from build123d import *

# Parameters (mm, degrees)
SKETCH1_W                    = 190
SKETCH1_H                    = 110
BASE_FLANGE1_DEPTH           = 1
EDGE_FLANGE1_START           = -72
EDGE_FLANGE1_DEPTH           = 144
EDGE_FLANGE2_STRIP_W         = 5.4732
EDGE_FLANGE2_STRIP_H         = 1
EDGE_FLANGE2_STRIP_CUT_DEPTH = 110
EDGE_FLANGE2_DEPTH           = 110
EDGE_FLANGE3_DEPTH           = 188.5268
SKETCH17_R                   = 2.25
SKETCH17_W                   = 10
SKETCH17_H                   = 25
CUT_EXTRUDE1_DEPTH           = 115.427372832
SKETCH18_R                   = 2.25
CUT_EXTRUDE2_DEPTH           = 115.427372832


# Read off the part's stored shape, not the designer's step: Edge-Flange1
# Sheet-metal steps are written as plain solids
with BuildPart() as part:
    # Sketch1 → Base-Flange1 (new body)
    with BuildSketch(Plane(origin=(0, 0, 0), x_dir=(1, 0, 0), z_dir=(0, 1, 0))):
        Rectangle(SKETCH1_W, SKETCH1_H)
    extrude(amount=-BASE_FLANGE1_DEPTH)

    # Edge-Flange1 outline → Edge-Flange1 (add)
    with BuildSketch(Plane.YZ.offset(EDGE_FLANGE1_START)):
        with BuildLine():
            Line((-11, -57.7366), (-1.7366, -57.7366))
            ThreePointArc((-1.7366, -57.7366), (-0.508638364, -57.227961636), (0, -56))
            Line((0, -56), (0, -55))
            Line((0, -55), (-1, -55))
            Line((-1, -55), (-1, -56))
            ThreePointArc((-1, -56), (-1.215745145, -56.520854855), (-1.7366, -56.7366))
            Line((-1.7366, -56.7366), (-11, -56.7366))
            Line((-11, -56.7366), (-11, -57.7366))
        make_face()
    extrude(amount=EDGE_FLANGE1_DEPTH)

    # Edge-Flange2 strip (across the edge) → Edge-Flange2 strip cut (cut)
    with BuildSketch(Plane(origin=(-95, -1, 55), x_dir=(1, 0, 0), z_dir=(0, 0, -1))):
        with Locations((-2, -0.5)):
            Rectangle(EDGE_FLANGE2_STRIP_W, EDGE_FLANGE2_STRIP_H)
    edge_flange2_strip_cut = extrude(amount=EDGE_FLANGE2_STRIP_CUT_DEPTH, mode=Mode.SUBTRACT)

    # Edge-Flange2 section (across the edge) → Edge-Flange2 (add)
    with BuildSketch(Plane(origin=(-95, -1, 55), x_dir=(1, 0, 0), z_dir=(0, 0, -1))):
        with BuildLine():
            Line((-1, 0.7366), (-1, 10))
            Line((-1, 10), (0, 10))
            Line((0, 10), (0, 0.7366))
            ThreePointArc((0, 0.7366), (0.215745145, 0.215745145), (0.7366, 0))
            Line((0.7366, 0), (0.7366, -1))
            ThreePointArc((0.7366, -1), (-0.491361636, -0.491361636), (-1, 0.7366))
        make_face()
    edge_flange2 = extrude(amount=EDGE_FLANGE2_DEPTH)

    # Mirror1: Edge-Flange2 strip cut, Edge-Flange2 across plane
    add(edge_flange2_strip_cut.mirror(Plane(origin=(0, 0, 0), x_dir=(0, 0, 1), z_dir=(1, 0, 0))), mode=Mode.SUBTRACT)
    add(edge_flange2.mirror(Plane(origin=(0, 0, 0), x_dir=(0, 0, 1), z_dir=(1, 0, 0))))

    # Edge-Flange3 section (across the edge) → Edge-Flange3 (add)
    with BuildSketch(Plane(origin=(94.2634, -1, 55.425276208), x_dir=(0, -0.5000000000000041, -0.8660254037844364), z_dir=(-1, 0, 0))):
        with BuildLine():
            Line((-1, 0.425276208), (-1, 10))
            Line((-1, 10), (0, 10))
            Line((0, 10), (0, 0.425276208))
            ThreePointArc((0, 0.425276208), (0.098685688, 0.056976208), (0.3683, -0.212638104))
            Line((0.3683, -0.212638104), (-0.1317, -1.078663508))
            ThreePointArc((-0.1317, -1.078663508), (-0.767339716, -0.443023792), (-1, 0.425276208))
        make_face()
    extrude(amount=EDGE_FLANGE3_DEPTH)

    # Sketch17 → Cut-Extrude1 (cut, through all)
    with BuildSketch(Plane(origin=(0, 0, 0), x_dir=(1, 0, 0), z_dir=(0, 1, 0))):
        with Locations(Location((66, 0, 0), (0, 0, 270))):
            Circle(SKETCH17_R)
        with Locations(Location((55, 0, 0), (0, 0, 270))):
            Circle(SKETCH17_R)
        with Locations(Location((-55, 0, 0), (0, 0, 270))):
            Circle(SKETCH17_R)
        with Locations(Location((-66, 0, 0), (0, 0, 270))):
            Circle(SKETCH17_R)
        with Locations((79, 0)):
            Rectangle(SKETCH17_W, SKETCH17_H)
        with Locations((-79, 0)):
            Rectangle(SKETCH17_W, SKETCH17_H)
    extrude(amount=-CUT_EXTRUDE1_DEPTH, mode=Mode.SUBTRACT)

    # Sketch18 → Cut-Extrude2 (cut, through all)
    with BuildSketch(Plane(origin=(0, 0, 0), x_dir=(1, 0, 0), z_dir=(0, 1, 0))):
        with Locations(Location((81.73, 50.2366, 0), (0, 0, 270))):
            Circle(SKETCH18_R)
        with Locations(Location((81.73, 39.2366, 0), (0, 0, 270))):
            Circle(SKETCH18_R)
        with Locations(Location((-81.73, 39.2366, 0), (0, 0, 270))):
            Circle(SKETCH18_R)
        with Locations(Location((-81.73, 50.2366, 0), (0, 0, 270))):
            Circle(SKETCH18_R)
    extrude(amount=-CUT_EXTRUDE2_DEPTH, mode=Mode.SUBTRACT)


solid = part.part
The listing builds one solid part. Answer for the finished solid, in the listing's coordinates (mm). A direction names the side the tool comes from. Round coordinates to 2 decimals unless told otherwise and drop trailing zeros. Write each loop counter-clockwise with the first axis right and the second up, starting at its lowest first coordinate (ties: lowest second). Pieces come first, ordered by that corner, then holes. Notation, with made-up numbers: (75.5, 18.5) - (114.5, 18.5) arc R25 cw to (114.5, 44.5) - close; hole circle Ø5 at (4.5, 55). An arc over 180 degrees is marked (long way). Use one line per item in the form item = value. Start each with the question number.
Item 1: A tool of negligible diameter and unlimited length cuts with its end or side. For faces 4 (the flat face through (-87.5, -0.6, -55)), 5 (the flat face through (87.5, -0.6, -55)), 6 (the flat face through (-95, -6, 1)), from which of +Z, -Z, +X, -X, +Y, -Y can it reach the whole face along a straight path? Write none if from no direction.
Item 2: Find the intervals of material crossed by line 1 (X direction, y = -3, z = 25.5); line 2 (Z direction, x = -21, y = -10.25); line 3 (Y direction, x = 73, z = -51), in increasing order. Write a range as [from, to].
Item 3: A cutting plane is placed at B-B (x = 81.73). Write down the section's boundary in (y, z).
Item 4: A cutting plane is placed at D-D (y = -6). Write down the section's boundary in (x, z), plus the area to 3 significant figures.
Item 5: A cutting plane is placed at C-C (z = 51). Write down the section's boundary in (x, y), plus the area to 3 significant figures.
Item 6: A cutting plane is placed at A-A (x = -55). Write down the section's boundary in (y, z), plus the area to 3 significant figures.
Item 7: Determine the mould class of faces 1 (the flat face through (-1, -1, -1)), 2 (the flat face through (-1, 0, -1)), 3 (the flat face through (-96, -6, 1)) for opening direction X: +X half, -X half, draft (parallel to the pull), parting line (faces both ways), or undercut.
Item 8: Flat-ended cylindrical pins translate along their axes: pin 1 Ø1.1 at (y, z) = (-0.5, 1) entering from +X; pin 2 Ø0.8 at (x, y) = (-77.5, -0.5) entering from -Z; pin 3 Ø5 at (x, z) = (-75.5, -0.5) entering from +Y; pin 4 Ø0.8 at (y, z) = (-0.5, -3.5) entering from -X. Find the tip coordinate at first contact, or state that the pin passes through.
The answers:
q1.face_4 = -Z, -X, +Y, -Y
q1.face_5 = -Z, +X, +Y, -Y
q1.face_6 = +Z, -Z, -Y
q2.line_1 = [-96, -95], [95, 96]
q2.line_2 = [-57.74, -56.74]
q2.line_3 = [-1, 0]
q3.outline = (-9.66, 60.43) - (-1.37, 55.64) arc R0.74 cw to (-1, 55) - (-1, 12.5) - (0, 12.5) - (0, 55) arc R1.74 ccw to (-0.87, 56.5) - (-9.16, 61.29) - close; (-1, -55) - (0, -55) - (0, -52.49) - (-1, -52.49) - close; (-1, -47.99) - (0, -47.99) - (0, -41.49) - (-1, -41.49) - close; (-1, -36.99) - (0, -36.99) - (0, -12.5) - (-1, -12.5) - close
q4.outline = (-96, -55) - (-95, -55) - (-95, 55) - (-96, 55) - close; (-94.26, 58.31) - (94.26, 58.31) - (94.26, 59.47) - (-94.26, 59.47) - close; (-72, -57.74) - (72, -57.74) - (72, -56.74) - (-72, -56.74) - close; (95, -55) - (96, -55) - (96, 55) - (95, 55) - close
q4.area = 582 mm^2
q5.outline = (-96, -11) - (-95, -11) - (-95, -1.74) arc R0.74 cw to (-94.26, -1) - (94.26, -1) arc R0.74 cw to (95, -1.74) - (95, -11) - (96, -11) - (96, -1.74) arc R1.74 ccw to (94.26, 0) - (-94.26, 0) arc R1.74 ccw to (-96, -1.74) - close
q5.area = 211 mm^2
q6.outline = (-11, -57.74) - (-1.74, -57.74) arc R1.74 ccw to (0, -56) - (0, -2.25) - (-1, -2.25) - (-1, -56) arc R0.74 cw to (-1.74, -56.74) - (-11, -56.74) - close; (-9.66, 60.43) - (-1.37, 55.64) arc R0.74 cw to (-1, 55) - (-1, 2.25) - (0, 2.25) - (0, 55) arc R1.74 ccw to (-0.87, 56.5) - (-9.16, 61.29) - close
q6.area = 129 mm^2
q7.face_1 = undercut
q7.face_2 = draft
q7.face_3 = -X half
q8.pin_1 = 95.86
q8.pin_2 = -55
q8.pin_3 = 0
q8.pin_4 = -95.79
